Source: three-view drawing plus pictorial views. Frame: mm from the lowest corner of the part. Coordinates: 2 decimals unless noted, no trailing zeros. Order: outer loops, then holes, each group sorted by start corner. A loop starts at its lowest first (then second) coordinate and runs counter-clockwise, first axis right, second up. Notation, with made-up numbers: (-34.5, -7) -> (18.5, -7) arc R20 cw to (18.5, 23) -> close; hole circle Ø10 at (77, -33). An arc over 180 degrees is marked (long way). One line per question, with ' | ' between items.
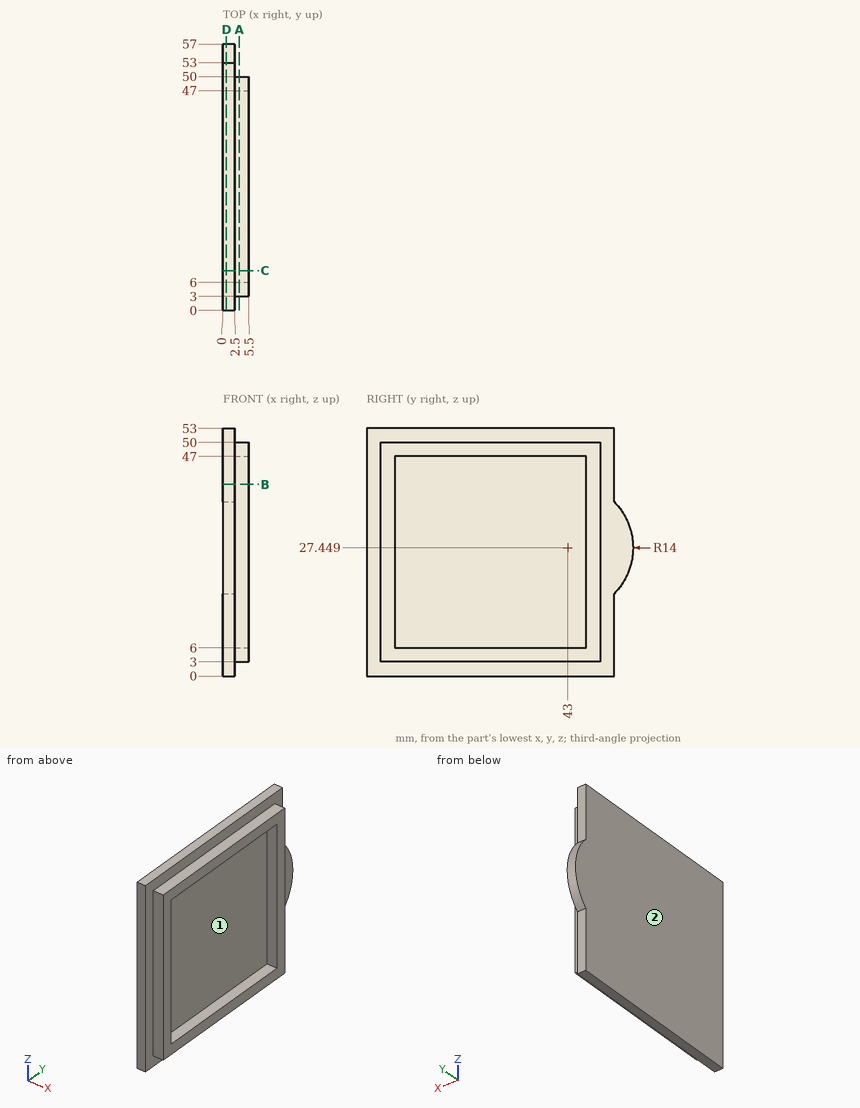
1. Cut plane A-A, the plane x = 3.5. Return loops of the section in (y, z), and give its area (3 significant figures).
Recorded:
outline: (3, 3) -> (50, 3) -> (50, 50) -> (3, 50) -> close; hole (6, 6) -> (47, 6) -> (47, 47) -> (6, 47) -> close | area: 528 mm^2
2. Pin query (flat end, axial travel): pin 1 Ø2 at (x, z) = (1.5, 4.5) entering from +Y; pin 2 Ø1.5 at (x, y) = (3.5, 30) entering from +Z; pin 3 Ø1.5 at (x, y) = (4.5, 15) entering from -Z. Return the tip coordinate at first contact, or that it passes through.
Recorded:
pin 1: stops at y = 53 | pin 2: stops at z = 50 | pin 3: stops at z = 3
3. Cut plane D-D, the plane x = 0.7. Return loops of the section in (y, z).
Recorded:
outline: (0, 0) -> (53, 0) -> (53, 17.65) arc R14 ccw to (53, 37.25) -> (53, 53) -> (0, 53) -> close
4. Ray query, line 1 (Y direction, x = 2.8, z = 18.5); line 2 (X direction, y = 21.5, z = 16). Return the intervals inside material, ascending. Write a range as [from, to].
Recorded:
line 1: y = [3, 6], [47, 50] | line 2: x = [0, 2.5]
5. Cut plane B-B, the plane z = 41. Return loops of the section in (x, y).
Recorded:
outline: (0, 0) -> (2.5, 0) -> (2.5, 3) -> (5.5, 3) -> (5.5, 6) -> (2.5, 6) -> (2.5, 47) -> (5.5, 47) -> (5.5, 50) -> (2.5, 50) -> (2.5, 53) -> (0, 53) -> close
6. Mould query, pull axis Z, two halves, no side actions, for the marked faces 1 and 2. Classes: released by +Z, released by -Z, zero draft, split by the parting line, or undercut.
Recorded:
face 1: undercut | face 2: zero draft
